from build123d import *

# Parameters (mm, degrees)
SKETCH1_R           = 1.5
SKETCH1_W           = 20
SKETCH1_H           = 3.2
BOSS_EXTRUDE1_DEPTH = 3
SKETCH2_W           = 3
SKETCH2_H           = 3.2
CUT_EXTRUDE1_DEPTH  = 10


with BuildPart() as part:
    # Sketch1 → Boss-Extrude1 (new body)
    with BuildSketch(Plane.XY):
        with BuildLine():
            Line((-45.069342458, 73), (29.930657542, 73))
            Line((29.930657542, 73), (29.930657542, 76))
            ThreePointArc((29.930657542, 76), (54.871173993, 78.743544354), (79.930657542, 80))
            Line((79.930657542, 80), (99.930657542, 80))
            Line((99.930657542, 80), (99.930657542, 73))
            ThreePointArc((99.930657542, 73), (99.94021491, 50.233693089), (98.469664685, 27.514927635))
            ThreePointArc((98.469664685, 27.514927635), (96.852910392, 24.29693628), (93.493249831, 23))
            Line((93.493249831, 23), (45.108726753, 23))
            ThreePointArc((45.108726753, 23), (43.13391621, 22.593487054), (41.480220087, 21.440049327))
            ThreePointArc((41.480220087, 21.440049327), (26.927174582, -0.016353332), (20, -25))
            Line((20, -25), (0, -25))
            Line((0, -25), (0, -27.9998915))
            Line((0, -27.9998915), (-20, -27.9998915))
            Line((-20, -27.9998915), (-20, -25))
            Line((-20, -25), (-99.408174518, -25))
            Line((-99.408174518, -25), (-90.591825482, 25))
            ThreePointArc((-90.591825482, 25), (-89.806825823, 27.489700841), (-88.404192383, 29.69139432))
            Line((-88.404192383, 29.69139432), (-56.560009105, 67.641814145))
            ThreePointArc((-56.560009105, 67.641814145), (-51.408616384, 71.594616806), (-45.069342458, 73))
        make_face()
        with Locations((69.930657542, 28)):
            Circle(SKETCH1_R, mode=Mode.SUBTRACT)
        with Locations((-15, 21.6)):
            Rectangle(SKETCH1_W, SKETCH1_H, mode=Mode.SUBTRACT)
        Polygon((-76.611843512, 39.077796972), (-74.160501294, 37.020876622), (-61.3047491, 52.341765484), (-63.756091318, 54.398685835), align=None, mode=Mode.SUBTRACT)
        Polygon((-93.782058518, -10.369022063), (-90.309094964, 9.327132997), (-87.157710155, 8.771458829), (-90.630673708, -10.924696232), align=None, mode=Mode.SUBTRACT)
    extrude(amount=BOSS_EXTRUDE1_DEPTH)

    # Sketch2 → Cut-Extrude1 (cut)
    with BuildSketch(Plane.XY.offset(3)):
        with Locations((98.430657542, 74.6)):
            Rectangle(SKETCH2_W, SKETCH2_H)
    extrude(amount=-CUT_EXTRUDE1_DEPTH, mode=Mode.SUBTRACT)


solid = part.part
Read the model definition and answer for the solid it produces. Units are mm, in the model's axes. A direction names the side the tool comes from. Round coordinates to 2 decimals unless told otherwise and drop trailing zeros. Loops run counter-clockwise (first coordinate to the right, second up) from the corner with the lowest first, then second, coordinate; pieces in that order, holes last. Notation, with made-up numbers: (11.5, 47) - (68.5, 47) arc R17 cw to (68.5, 70) - close; hole circle Ø5 at (46.5, 8.25). An arc over 180 degrees is marked (long way). One line per question, with ' | ' between items. Start each with the question number.
Q1. For a pull along Y with two mould halves and no side action, classify faces 3 (the flat face through (2, 27, 3)), 4 (the flat face through (-92.07, -0.66, 1.48)), 5 (the cylindrical face through (27.08, 0.31, 1.48)) as +Y half, -Y half, draft (parallel to the pull), parting line (faces both ways), or undercut.
Q2. Section A-A on y = 6.5 is taken. Give the vertices of the cut face in (x, z), plus the area to 3 significant figures.
Q3. Section B-B on z = 2.1 is taken. Count the separate pieces of the cut face and the enclosed holes in it, plus the area to 3 significant figures.
Q4. Find the intervals of material crossed by L1, parallel to Y at x = 5, z = 0.9; L2, parallel to Y at x = 78, z = 0.35; L3, parallel to X at y = 3, z = 1.3, in increasing order.
Q5. Flat-ended cylindrical pins translate along their axes: pin 1 (1.5 mm diameter, centred on y = 75.5, z = 1, fed in from +X); pin 2 (1.5 mm diameter, centred on y = -27, z = 2, fed in from -X); pin 3 (1.5 mm diameter, centred on x = 98, z = 1.5, fed in from -Y). Find the tip coordinate at first contact, or state that the pin passes through.
Q6. Section C-C on x = 14.5 is taken. Give the vertices of the cut face in (y, z), plus the area to 3 significant figures.
Q7. For faces 1 (the cylindrical face through (96.89, 24.33, 1.48)), 2 (the flat face through (-88.87, -0.94, 1.48)), determine the directions among +Z, -Z, +X, -X, +Y, -Y from which every point of the face is accessible in a straight line to the end or side of a thin tool.
Q8. Section D-D on y = -19 is taken. Give the vertices of the cut face in (x, z).
Established:
1) face 3: draft | face 4: undercut | face 5: -Y half
2) outline: (-93.85, 0) - (-90.81, 0) - (-90.81, 3) - (-93.85, 3) - close; (-87.56, 0) - (30.31, 0) - (30.31, 3) - (-87.56, 3) - close | area: 363 mm²
3) separate pieces: 1 | enclosed holes: 4 | area: 14,800 mm²
4) L1: -25 to 73 | L2: 23 to 79.96 | L3: -94.47 to -91.42, -88.18 to 28.4
5) pin 1: x = 99.93 | pin 2: x = -20 | pin 3: y = 24.7
6) outline: (-25, 0) - (73, 0) - (73, 3) - (-25, 3) - close | area: 294 mm²
7) face 1: +Z, -Z, +X, -Y | face 2: +Z, -Z
8) outline: (-98.35, 0) - (20.88, 0) - (20.88, 3) - (-98.35, 3) - close
